Check sheet for the modelled part. Datum: model origin and axes. Units: mm. Round coordinates to 2 decimals unless told otherwise and drop trailing zeros. Write each loop counter-clockwise with the first axis right and the second up, starting at its lowest first coordinate (ties: lowest second). Pieces come first, ordered by that corner, then holes. Notation, with made-up numbers: (62, 68.5) -> (112, 68.5) arc R25 ccw to (112, 86.5) -> close; hole circle Ø2 at (-9, 19.25). An arc over 180 degrees is marked (long way). Put each result on its own line as item: value. Start each with the question number.
Autodesk Inventor part; units mm, degrees
ref_plane "YZ Plane" through (0, 0, 0) normal (1, 0, 0) x (0, 1, 0)
ref_plane "XZ Plane" through (0, 0, 0) normal (0, 1, 0) x (-1, 0, 0)
ref_plane "XY Plane" through (0, 0, 0) normal (0, 0, 1) x (1, 0, 0)
sketch "Sketch1" plane through (0, 0, 0) normal (0, 0, 1) x (1, 0, 0)
  line L0 (0, 0) -> (228.6, 0)
  line L1 (228.6, 0) -> (228.6, 127)
  line L2 (228.6, 127) -> (0, 127)
  line L3 (0, 127) -> (0, 0)
  dimension "d0" = 228.6
  dimension "d1" = 127
extrude "Extrusion1" add sketch "Sketch1" against normal blind 3.175
sketch "Sketch2" plane through (0, 0, 0) normal (0, 0, 1) x (1, 0, 0)
  line L0 (0, 0) -> (228.6, 0)
  line L1 (0, 127) -> (0, 0)
  point P0 (38.1, 31.75)
  point P1 (76.2, 31.75)
  point P2 (116.9154, 31.75)
  point P3 (157.6309, 31.75)
  point P4 (198.3463, 31.75)
  point P5 (0, 63.5)
  dimension "d4" = 31.75
  dimension "d5" = 38.1
  dimension "d6" = 38.1
  dimension "d7" = 40.7154
  dimension "d8" = 40.7154
  dimension "d9" = 40.7154
hole "Hole1" at (38.1, 31.75, 0) direction (0, 0, -1) diameter 28.2956 end through all
hole "Hole2" at (76.2, 31.75, 0) direction (0, 0, -1) diameter 28.321 end through all
hole "Hole3" at (116.9154, 31.75, 0) direction (0, 0, -1) diameter 28.3464 end through all
hole "Hole4" at (157.6309, 31.75, 0) direction (0, 0, -1) diameter 28.3718 end through all
hole "Hole5" at (198.3463, 31.75, 0) direction (0, 0, -1) diameter 28.3972 end through all
sketch "Sketch3" plane through (0, 0, 0) normal (0, 0, 1) x (1, 0, 0)
  line L0 (0, 0) -> (0, 127) construction
  line L1 (0, 63.5) -> (228.6, 63.5) construction
  line L2 (228.6, 127) -> (228.6, 0) construction
  point P0 (38.1, 31.75)
  point P1 (76.2, 31.75)
  point P2 (116.9154, 31.75)
  point P3 (157.6309, 31.75)
  point P4 (198.3463, 31.75)
  point P5 (38.1, 95.25)
  point P6 (76.2, 95.25)
  point P7 (116.9154, 95.25)
  point P8 (157.6309, 95.25)
  point P9 (198.3463, 95.25)
hole "Hole6" at (38.1, 95.25, 0) direction (0, 0, -1) diameter 21.971 end through all
hole "Hole7" at (76.2, 95.25, 0) direction (0, 0, -1) diameter 21.971 end through all
hole "Hole8" at (116.9154, 95.25, 0) direction (0, 0, -1) diameter 21.9964 end through all
hole "Hole9" at (157.6309, 95.25, 0) direction (0, 0, -1) diameter 22.0218 end through all
hole "Hole10" at (198.3463, 95.25, 0) direction (0, 0, -1) diameter 22.0472 end through all
properties part number "BEARING TEST" material "Aluminum 6061"
1. Material ranges on L1, parallel to X at y = 95.25, z = -0.65; L2, parallel to Y at x = 76.2, z = -1; L3, parallel to Y at x = 154.5, z = -0.95, recorded low to high. Write a range as [from, to].
2. Section check B-B, the plane x = 76.2. Enter the section's corners in (y, z) (1 decimal).
3. Section check A-A, the plane y = 95.25. Enter the section's corners in (x, z) (1 decimal).
4. Section check D-D, the plane y = 31.75. Enter the section's corners in (x, z) (1 decimal).
5. Draft check along X on faces 1 (the flat face through (113, 64, -3.175)), 2 (the cylindrical face through (109.482, 103.356, -1.61)). Enter one of: released by +X, released by -X, zero draft, split by the parting line, or undercut.
6. Section check C-C, the plane z = -0.8. Give the number of separate pieces and of enclosed holes in the cut face, then the cut area to 3 significant figures.
Reply:
1. L1: x = [0, 27.11], [49.09, 65.21], [87.19, 105.92], [127.91, 146.62], [168.64, 187.32], [209.37, 228.6]
1. L2: y = [0, 17.59], [45.91, 84.26], [106.24, 127]
1. L3: y = [0, 17.91], [45.59, 84.69], [105.81, 127]
2. outline: (0, -3.2) -> (17.6, -3.2) -> (17.6, 0) -> (0, 0) -> close; (45.9, -3.2) -> (84.3, -3.2) -> (84.3, 0) -> (45.9, 0) -> close; (106.2, -3.2) -> (127, -3.2) -> (127, 0) -> (106.2, 0) -> close
3. outline: (0, -3.2) -> (27.1, -3.2) -> (27.1, 0) -> (0, 0) -> close; (49.1, -3.2) -> (65.2, -3.2) -> (65.2, 0) -> (49.1, 0) -> close; (87.2, -3.2) -> (105.9, -3.2) -> (105.9, 0) -> (87.2, 0) -> close; (127.9, -3.2) -> (146.6, -3.2) -> (146.6, 0) -> (127.9, 0) -> close; (168.6, -3.2) -> (187.3, -3.2) -> (187.3, 0) -> (168.6, 0) -> close; (209.4, -3.2) -> (228.6, -3.2) -> (228.6, 0) -> (209.4, 0) -> close
4. outline: (0, -3.2) -> (24, -3.2) -> (24, 0) -> (0, 0) -> close; (52.2, -3.2) -> (62, -3.2) -> (62, 0) -> (52.2, 0) -> close; (90.4, -3.2) -> (102.7, -3.2) -> (102.7, 0) -> (90.4, 0) -> close; (131.1, -3.2) -> (143.4, -3.2) -> (143.4, 0) -> (131.1, 0) -> close; (171.8, -3.2) -> (184.1, -3.2) -> (184.1, 0) -> (171.8, 0) -> close; (212.5, -3.2) -> (228.6, -3.2) -> (228.6, 0) -> (212.5, 0) -> close
5. face 1: zero draft
5. face 2: undercut
6. separate pieces: 1
6. enclosed holes: 10
6. area: 24,000 mm2
